For this review, take the finished solid that the model builds, in its own axes (mm). A direction names the side the tool comes from. Round coordinates to 2 decimals unless told otherwise and drop trailing zeros. Loops run counter-clockwise (first coordinate to the right, second up) from the corner with the lowest first, then second, coordinate; pieces in that order, holes last. Notation, with made-up numbers: (-11.5, 63) -> (31.5, 63) arc R14 cw to (31.5, 77) -> close; hole circle Ø2 at (-32.75, 30.5). An arc over 180 degrees is marked (long way). One line per question, with ' | ' between items. Start each with the question number.
1. For faces 4 (the face through (-5.992, -1.742, 5.532)), 5 (the face through (7.817, -1.802, 5.723)), list the 3-axis set-ups (+Z, -Z, +X, -X, +Y, -Y) from which the entire face can be reached by the end or side of a thin tool; tool diameter is ignored.
2. For pin 1 Ø1 at (x, y) = (-4.5, -1.5) entering from +Z; pin 2 Ø6 at (x, z) = (5, -4) entering from +Y, all flat-tipped, find the tip position at first contact; note any pin that passes through.
3. Consider section D-D (x = -2.75). Write out the cut boundary in (y, z), and give its area (3 significant figures).
4. Wall thickness on line 1 along Y through (x, z) = (3.75, 0); line 2 along Y through (x, z) = (-6, 2.5); line 3 along Z through (x, y) = (-4.25, -2): over which ranges is each line inside the solid? List them lowest first.
5. Consider section C-C (x = 5.75). Write out the cut boundary in (y, z), and give its area (3 significant figures).
6. Draft analysis for pull direction Z (two halves, no side actions). For faces 1 (the face through (6.008, -1.742, 5.532)), 2 (the face through (-0.13, -0.9, 2.86)), 3 (the face through (-9.5, 2.4, -2.4)), state which applies: pulls with the +Z half, pulls with the -Z half, needs draft (parallel to the pull), parting line crosses it, or undercut.
7. Consider section A-A (z = 0). Write out the cut boundary in (x, y).
```python
from build123d import *

# Parameters (mm, degrees)
FILLET1_R = 0.5


with BuildPart() as part:
    # Sketch2 → Revolve1 (revolve)
    with BuildSketch(Plane(origin=(0, 0, 0), x_dir=(1, 0, 0), z_dir=(0, 1, 0)), mode=Mode.PRIVATE) as revolve1_sk:
        Polygon((-5.4, 6), (5.4, 6), (5.4, 5.8), (6.6, 5.8), (6.6, 6), (9.5, 6), (9.5, 3), (-9.5, 3), (-9.5, 6), (-6.6, 6), (-6.6, 5.8), (-5.4, 5.8), align=None)
    revolve(revolve1_sk.sketch.rotate(Axis((0, 0, 0), (1, 0, 0)), 180), axis=Axis((0, 0, 0), (1, 0, 0)))

    # Fillet1
    fillet1_edges = [part.edges().sort_by_distance(p)[0] for p in [
        (-9.5, 0, -6),
        (9.5, 0, -6),
    ]]
    fillet(fillet1_edges, radius=FILLET1_R)


solid = part.part
```
Answer block:
1) face 4: none | face 5: +X, -X
2) pin 1: stops at z = 5.92 | pin 2: stops at y = 5.92
3) outline: circle Ø12 at (0, 0); hole circle Ø6 at (0, 0) | area: 84.8 mm2
4) line 1: y = -6 to -3, 3 to 6 | line 2: y = -5.23 to -1.66, 1.66 to 5.23 | line 3: z = -5.66 to -2.24, 2.24 to 5.66
5) outline: circle Ø11.6 at (0, 0); hole circle Ø6 at (0, 0) | area: 77.4 mm2
6) face 1: parting line crosses it | face 2: undercut | face 3: needs draft
7) outline: (-9.5, -5.5) arc R0.5 ccw to (-9, -6) -> (-6.6, -6) -> (-6.6, -5.8) -> (-5.4, -5.8) -> (-5.4, -6) -> (5.4, -6) -> (5.4, -5.8) -> (6.6, -5.8) -> (6.6, -6) -> (9, -6) arc R0.5 ccw to (9.5, -5.5) -> (9.5, -3) -> (-9.5, -3) -> close; (-9.5, 3) -> (9.5, 3) -> (9.5, 5.5) arc R0.5 ccw to (9, 6) -> (6.6, 6) -> (6.6, 5.8) -> (5.4, 5.8) -> (5.4, 6) -> (-5.4, 6) -> (-5.4, 5.8) -> (-6.6, 5.8) -> (-6.6, 6) -> (-9, 6) arc R0.5 ccw to (-9.5, 5.5) -> close
